Geometry check sheet. Reference: the model listing, model coordinates, mm. A direction names the side the tool comes from. Round coordinates to 2 decimals unless told otherwise and drop trailing zeros. Write each loop counter-clockwise with the first axis right and the second up, starting at its lowest first coordinate (ties: lowest second). Pieces come first, ordered by that corner, then holes. Notation, with made-up numbers: M 55.25,32.5 L 74.25,32.5 A13 cw 74.25,54.5 Z; hole C 44,-39 d1. An arc over 180 degrees is marked long. One line per item, written item: value. Start each with the question number.
1. Section check D-D (y = 33). Record the boundary of the cut face in (x, z), and give its area (3 significant figures).
2. Access from +Z, -Z, +X, -X, +Y, -Y to the whole of each face (thin tool, end or side, straight path). Record for faces 5 (the cylindrical face through (-13.743, 52.172, 2.958)), 6 (the flat face through (9, 5, 3)).
3. Release check for a two-part mould opening along X. For faces 1 (the flat face through (-6, 28.348, 5)), 2 (the cylindrical face through (-2.17, -9.76, 1.48)), 3 (the flat face through (-7.5, 41.8, 3.9)), 4 (the flat face through (-8.9, 53.8, 2.3)) record: pulls with the +X half, pulls with the -X half, needs draft (parallel to the pull), parting line crosses it, or undercut.
4. Section check A-A (x = 0). Record the boundary of the cut face in (y, z), and give its area (3 significant figures).
5. Section check B-B (y = 8.5). Record the boundary of the cut face in (x, z), and give its area (3 significant figures).
6. Depth check by flat-ended pin: P1, Ø12, axis at x = 0, y = 0, coming from the +Z side (3 decimals); P2, Ø3, axis at y = 12.5, z = 1.5, coming from the -X side; P3, Ø1.1, axis at x = -7.5, z = 4, coming from the +Y side; P4, Ø21, axis at x = 6.5, y = -0.5, coming from the +Z side. Enter the tip coordinate at first touch or a pass-through.
7. Scan lines: probe 1 along Z at (x, y) = (-14.5, -7.5); probe 2 along Y at (x, z) = (0, 1); probe 3 along Y at (x, z) = (8.5, 1.4). Record each from-to range of solid material in increasing order. Write a range as [from, to].
8. Section check C-C (z = 0.7). Record the boundary of the cut face in (x, y).
from build123d import *

# Parameters (mm, degrees)
CROQUIS1_R                = 10
SALIENTE_EXTRUIR1_DEPTH   = 6
CROQUIS2_R                = 21
CROQUIS2_R_2              = 10
CORTAR_EXTRUIR1_DEPTH     = 3
CORTAR_EXTRUIR2_DEPTH     = 26
REDONDEO1_R               = 0.5
TALADRO_ROSCADO_M51_D     = 4.2
TALADRO_ROSCADO_M51_DEPTH = 14
TALADRO_ROSCADO_M51_TIP   = 1.2618073


with BuildPart() as part:
    # Croquis1 → Saliente-Extruir1 (new body)
    with BuildSketch(Plane.XY):
        with BuildLine():
            Line((-16.7, 12.732242536), (-14.762225987, 49.707173354))
            ThreePointArc((-14.762225987, 49.707173354), (-13.716817195, 52.20019036), (-11.324400252, 53.458901804))
            Line((-11.324400252, 53.458901804), (-5, 54.347738295))
            Line((-5, 54.347738295), (-5, 20.396078054))
            ThreePointArc((-5, 20.396078054), (11.506784682, -17.566841102), (-16.7, 12.732242536))
        make_face()
        Circle(CROQUIS1_R, mode=Mode.SUBTRACT)
    extrude(amount=SALIENTE_EXTRUIR1_DEPTH)

    # Croquis2 → Cortar-Extruir1 (cut)
    with BuildSketch(Plane.XY.offset(6)):
        Circle(CROQUIS2_R)
        Circle(CROQUIS2_R_2, mode=Mode.SUBTRACT)
    extrude(amount=-CORTAR_EXTRUIR1_DEPTH, mode=Mode.SUBTRACT)

    # Croquis3 → Cortar-Extruir2 (cut)
    with BuildSketch(Plane(origin=(0, 54.347738295, 0), x_dir=(-1, 0, 0), z_dir=(0, 1, 0))):
        Polygon((10.005365089, 6), (5, 1.8), (5, 6), align=None)
    extrude(amount=-CORTAR_EXTRUIR2_DEPTH, mode=Mode.SUBTRACT)

    # Redondeo1
    redondeo1_edges = [part.edges().sort_by_distance(p)[0] for p in [
        (-7.502682544, 28.347738295, 3.9),
    ]]
    fillet(redondeo1_edges, radius=REDONDEO1_R)

    # Taladro roscado M51
    with Locations(Plane.XY.offset(6)):
        with Locations((-10, 23)):
            Hole(TALADRO_ROSCADO_M51_D / 2, depth=TALADRO_ROSCADO_M51_DEPTH)
            with Locations((0, 0, -(TALADRO_ROSCADO_M51_DEPTH + TALADRO_ROSCADO_M51_TIP / 2))):  # 118° drill point
                Cone(0, TALADRO_ROSCADO_M51_D / 2, TALADRO_ROSCADO_M51_TIP, mode=Mode.SUBTRACT)


solid = part.part
Result sheet:
1. outline: M -15.64,0 L -5,0 L -5,1.8 L -10.01,6 L -15.64,6 Z
1. area: 53.3 mm2
2. face 5: +Z, -Z, -X, +Y
2. face 6: +Z, +X, -Y
3. face 1: needs draft
3. face 2: undercut
3. face 3: pulls with the +X half
3. face 4: pulls with the -X half
4. outline: M -21,0 L -10,0 L -10,3 L -21,3 Z; M 10,0 L 21,0 L 21,3 L 10,3 Z
4. area: 66.0 mm2
5. outline: M -19.2,0 L -5.27,0 L -5.27,3 L -19.2,3 Z; M 5.27,0 L 19.2,0 L 19.2,3 L 5.27,3 Z
5. area: 83.6 mm2
6. P1: passes through
6. P2: stops at x = -17.89
6. P3: stops at y = 54.05
6. P4: stops at z = 3
7. probe 1: z = [0, 3]
7. probe 2: y = [-21, -10], [10, 21]
7. probe 3: y = [-19.2, -5.27], [5.27, 19.2]
8. outline: M -16.7,12.73 A21 ccw long -5,20.4 L -5,54.35 L -11.32,53.46 A4 ccw -14.76,49.71 Z; hole C -10,23 d4.2; hole C 0,0 d20
